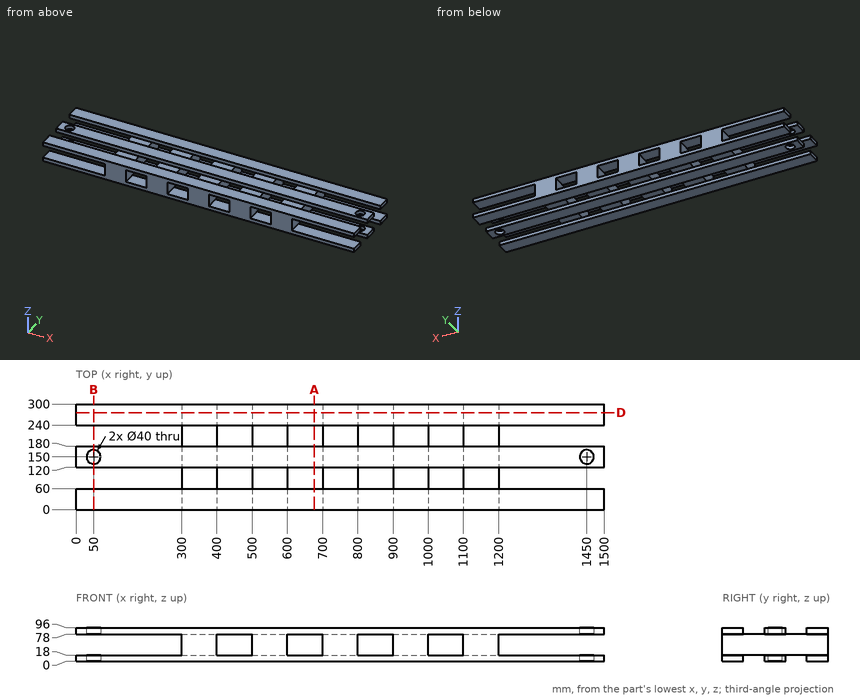
Verification items for this drawing (mm, ordinates from the low corner). Give positions to 0.01 mm unless a question says otherwise; leave off trailing zeros. Loops run counter-clockwise (first coordinate to the right, second up) from the corner with the lowest first, then second, coordinate; pieces in that order, holes last. Notation, with made-up numbers: (45, -24) - (71, -24) arc R19 cw to (71, -5) - close; hole circle Ø1 at (15.25, 20.5). An arc over 180 degrees is marked (long way). Write item = value, one per line. Start each with the question number.
Q1. Cross-section at A-A, the plane x = 677. Enter the section's corners in (y, z), and give its area (3 significant figures).
Q2. Thickness scan on line 1 (Y direction, x = 50, z = 86.25); line 2 (X direction, y = 162.5, z = 33); line 3 (Y direction, x = 62.5, z = 79). Record the ranges inside material, lowest first.
Q3. Depth check by flat-ended pin: P1, Ø18, axis at x = 1135, y = 76, coming from the +Z side; P2, Ø4, axis at y = 106.5, z = 48.5, coming from the +X side; P3, Ø1, axis at y = 151, z = 43, coming from the -X side; P4, Ø4, axis at x = 404, z = 18, coming from the -Y side. Enter the tip coordinate at first touch or a pass-through.
Q4. Cross-section at D-D, the plane y = 275.5. Enter the section's corners in (x, z).
Q5. Cross-section at B-B, the plane x = 50. State how many separate pieces and enclosed holes the cut face has, and give its area (3 significant figures).
Answer key:
q1.outline = (0, 0) - (60, 0) - (60, 18) - (0, 18) - close; (0, 78) - (60, 78) - (60, 96) - (0, 96) - close; (120, 0) - (180, 0) - (180, 18) - (120, 18) - close; (120, 78) - (180, 78) - (180, 96) - (120, 96) - close; (240, 0) - (300, 0) - (300, 18) - (240, 18) - close; (240, 78) - (300, 78) - (300, 96) - (240, 96) - close
q1.area = 6,480 mm^2
q2.line_1 = 0 to 60, 120 to 130, 170 to 180, 240 to 300
q2.line_2 = 300 to 400, 500 to 600, 700 to 800, 900 to 1000, 1100 to 1200
q2.line_3 = 0 to 60, 120 to 134.39, 165.61 to 180, 240 to 300
q3.P1 = 78
q3.P2 = 1200
q3.P3 = 300
q3.P4 = 0
q4.outline = (0, 0) - (1500, 0) - (1500, 18) - (1200, 18) - (1200, 78) - (1500, 78) - (1500, 96) - (0, 96) - (0, 78) - (300, 78) - (300, 18) - (0, 18) - close; hole (400, 18) - (500, 18) - (500, 78) - (400, 78) - close; hole (600, 18) - (700, 18) - (700, 78) - (600, 78) - close; hole (800, 18) - (900, 18) - (900, 78) - (800, 78) - close; hole (1000, 18) - (1100, 18) - (1100, 78) - (1000, 78) - close
q5.separate_pieces = 8
q5.enclosed_holes = 0
q5.area = 5,040 mm^2
